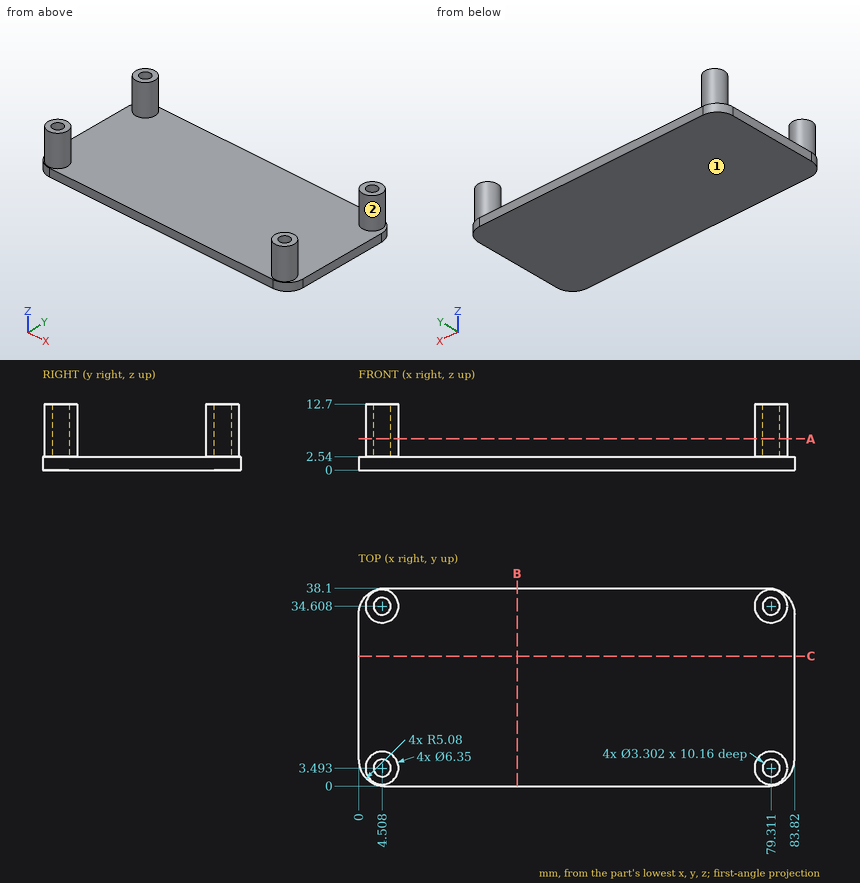
Part print with two shaded views. Sizes in mm from the minimum x, y, z corner. Round coordinates to 2 decimals unless told otherwise and drop trailing zeros. Loops run counter-clockwise (first coordinate to the right, second up) from the corner with the lowest first, then second, coordinate; pieces in that order, holes last. Notation, with made-up numbers: M -9,88.25 L 38,88.25 A18 ccw 38,105.25 Z; hole C -39,89.25 d2. An arc over 180 degrees is marked long. Put each result on its own line as item: value. Start each with the question number.
Item 1: Drill centre lines: line 1 along X through (y, z) = (36, 3.25) (1 decimal); line 2 along X through (y, z) = (34, 12) (1 decimal); line 3 along Y through (x, z) = (6, 4) (1 decimal). Where is each one in solid material? Low to high.
Item 2: Cut at C-C (y = 25). List the corners of the cut face in (x, z), then the cut area to 3 significant figures.
Item 3: Cut at A-A (z = 6). Give the number of separate pieces and of enclosed holes in the cut face.
Item 4: Cut at B-B (x = 30.5). List the corners of the cut face in (y, z).
Item 5: Mould opens along X. For the marked faces 1 and 2 say: released by +X, released by -X, zero draft, split by the parting line, or undercut.
Item 6: Drop flat-ended pins along their axis: P1, Ø1, axis at x = 79, y = 35.5, coming from the +Z side; P2, Ø2, axis at x = 79.31, y = 3.49, coming from the -Z side. Give the stop position or say it passes through.
Answer block:
1. line 1: 1.7 to 3.6, 5.4 to 7.4, 76.5 to 78.4, 80.2 to 82.2
1. line 2: 1.4 to 3, 6 to 7.6, 76.2 to 77.8, 80.8 to 82.4
1. line 3: 0.7 to 2.8, 4.2 to 6.3, 31.8 to 33.9, 35.3 to 37.4
2. outline: M 0,0 L 83.82,0 L 83.82,2.54 L 0,2.54 Z
2. area: 213 mm2
3. separate pieces: 4
3. enclosed holes: 4
4. outline: M 0,0 L 38.1,0 L 38.1,2.54 L 0,2.54 Z
5. face 1: zero draft
5. face 2: undercut
6. P1: z = 2.54
6. P2: z = 0
